from build123d import *
from OCP.BRepFilletAPI import BRepFilletAPI_MakeChamfer

# Parameters (mm, degrees)
EXTRUDE_1_DEPTH    = 2.4
HOLE_WIZARD_M3_1_D = 3.242
CHAMFER_1_SIZE     = 0.45
CHAMFER_1_SIZE_2   = 0.259807621
CHAMFER_3_SIZE     = 0.379


with BuildPart() as part:
    # 草圖1 → 填料-伸長1 (new body)
    with BuildSketch(Plane(origin=(0, 0, 0), x_dir=(0, -1, 0), z_dir=(-1, 0, 0))):
        with BuildLine():
            Line((-1.746239959, 2.975423668), (-3.449912463, 0.024576332))
            ThreePointArc((-3.449912463, 0.024576332), (-3.45, 0), (-3.449912463, -0.024576332))
            Line((-3.449912463, -0.024576332), (-1.746239959, -2.975423668))
            ThreePointArc((-1.746239959, -2.975423668), (-1.725, -2.987787643), (-1.703672504, -3))
            Line((-1.703672504, -3), (1.703672504, -3))
            ThreePointArc((1.703672504, -3), (1.725, -2.987787643), (1.746239959, -2.975423668))
            Line((1.746239959, -2.975423668), (3.449912463, -0.024576332))
            ThreePointArc((3.449912463, -0.024576332), (3.45, 0), (3.449912463, 0.024576332))
            Line((3.449912463, 0.024576332), (1.746239959, 2.975423668))
            ThreePointArc((1.746239959, 2.975423668), (1.725, 2.987787643), (1.703672504, 3))
            Line((1.703672504, 3), (-1.703672504, 3))
            ThreePointArc((-1.703672504, 3), (-1.725, 2.987787643), (-1.746239959, 2.975423668))
        make_face()
    extrude(amount=-EXTRUDE_1_DEPTH)

    # M3 餘隙孔1 (through all)
    with Locations(Plane(origin=(2.4, 0, 0), x_dir=(0, 0, -1), z_dir=(1, 0, 0))):
        with Locations((0, 0)):
            Hole(HOLE_WIZARD_M3_1_D / 2)

    # 導角1
    chamfer_1_edges_1 = [part.edges().sort_by_distance(p)[0] for p in [
        (0, -3.45, 0),
    ]]
    chamfer_1_side_1 = [part.faces().sort_by_distance(p)[0] for p in [
        (0, -3.444803848, 0),
    ]]
    chamfer_1_edges_2 = [part.edges().sort_by_distance(p)[0] for p in [
        (0, 1.725, 2.987787643),
    ]]
    chamfer_1_side_2 = [part.faces().sort_by_distance(p)[0] for p in [
        (0.005196152, 1.725, 2.987787643),
    ]]
    chamfer_1_edges_3 = [part.edges().sort_by_distance(p)[0] for p in [
        (0, 3.45, 0),
    ]]
    chamfer_1_side_3 = [part.faces().sort_by_distance(p)[0] for p in [
        (0, 3.444803848, 0),
    ]]
    chamfer_1_edges_4 = [part.edges().sort_by_distance(p)[0] for p in [
        (0, 1.725, -2.987787643),
    ]]
    chamfer_1_side_4 = [part.faces().sort_by_distance(p)[0] for p in [
        (0, 1.722401924, -2.983287643),
    ]]
    chamfer_1_edges_5 = [part.edges().sort_by_distance(p)[0] for p in [
        (0, -1.725, -2.987787643),
    ]]
    chamfer_1_side_5 = [part.faces().sort_by_distance(p)[0] for p in [
        (0, -1.722401924, -2.983287643),
    ]]
    chamfer_1_edges_6 = [part.edges().sort_by_distance(p)[0] for p in [
        (2.4, -1.725, 2.987787643),
    ]]
    chamfer_1_side_6 = [part.faces().sort_by_distance(p)[0] for p in [
        (2.4, -1.722401924, 2.983287643),
    ]]
    chamfer_1_edges_7 = [part.edges().sort_by_distance(p)[0] for p in [
        (2.4, 3.45, 0),
    ]]
    chamfer_1_side_7 = [part.faces().sort_by_distance(p)[0] for p in [
        (2.4, 3.444803848, 0),
    ]]
    chamfer_1 = BRepFilletAPI_MakeChamfer(part.part.solid().wrapped)
    for e in chamfer_1_edges_1:
        chamfer_1.Add(CHAMFER_1_SIZE - 0.0001, CHAMFER_1_SIZE_2 - 0.0001, e.wrapped, chamfer_1_side_1[0].wrapped)
    for e in chamfer_1_edges_2:
        chamfer_1.Add(CHAMFER_1_SIZE_2 - 0.0001, CHAMFER_1_SIZE - 0.0001, e.wrapped, chamfer_1_side_2[0].wrapped)
    for e in chamfer_1_edges_3:
        chamfer_1.Add(CHAMFER_1_SIZE - 0.0001, CHAMFER_1_SIZE_2 - 0.0001, e.wrapped, chamfer_1_side_3[0].wrapped)
    for e in chamfer_1_edges_4:
        chamfer_1.Add(CHAMFER_1_SIZE - 0.0001, CHAMFER_1_SIZE_2 - 0.0001, e.wrapped, chamfer_1_side_4[0].wrapped)
    for e in chamfer_1_edges_5:
        chamfer_1.Add(CHAMFER_1_SIZE - 0.0001, CHAMFER_1_SIZE_2 - 0.0001, e.wrapped, chamfer_1_side_5[0].wrapped)
    for e in chamfer_1_edges_6:
        chamfer_1.Add(CHAMFER_1_SIZE_2 - 0.0001, CHAMFER_1_SIZE - 0.0001, e.wrapped, chamfer_1_side_6[0].wrapped)
    for e in chamfer_1_edges_7:
        chamfer_1.Add(CHAMFER_1_SIZE_2 - 0.0001, CHAMFER_1_SIZE - 0.0001, e.wrapped, chamfer_1_side_7[0].wrapped)
    add(Compound.cast(chamfer_1.Shape()), mode=Mode.REPLACE)  # a hair under: the kernel refuses the full size

    # 導角3
    chamfer_3_edges = [part.edges().sort_by_distance(p)[0] for p in [
        (2.4, 0, -1.621),
        (0, 0, -1.621),
    ]]
    chamfer(chamfer_3_edges, length=CHAMFER_3_SIZE)


solid = part.part
Geometry: final body of the model. Coordinates: model frame, mm. Round coordinates to 2 decimals unless told otherwise and drop trailing zeros. Loops run counter-clockwise (first coordinate to the right, second up) from the corner with the lowest first, then second, coordinate; pieces in that order, holes last. Notation, with made-up numbers: M -0.75,29 L 24.25,29 A25 ccw 24.25,47 Z; hole C 33,43 d9. An arc over 180 degrees is marked long. Put each result on its own line as item: value. Start each with the question number.
(1) Contact query for flat-ended pins moving along their axis: pin 1 Ø1 at (x, z) = (2, 2.5) entering from -Y; pin 2 Ø1 at (x, y) = (1, -2.5) entering from +Z; pin 3 Ø2.5 at (y, z) = (0, 0) entering from +X. Output: stop coordinate, or through.
(2) Draft query along Y for faces 1 (the face through (1, 0, 3)), 2 (the face through (1.189, -1.438, 0.748)), 3 (the face through (0.102, -3.176, -0.008)). Return one class per face: +Y half, -Y half, draft (parallel to the pull), parting line (faces both ways), or undercut.
(3) Material intervals for line 1 along Y through (x, z) = (1.35, 0); line 2 along Y through (x, z) = (0.95, 1.4); line 3 along Z through (x, y) = (1.7, 2.25), sorted ascending. Write a range as [from, to].
(4) Section query A-A (x = 1.85). Return loops of the section in (y, z).
(5) Section query B-B (x = 2.2). Return loops of the section in (y, z), then the cut area to 3 significant figures.
Findings below:
1. pin 1: stops at y = -2.31
1. pin 2: stops at z = 2.54
1. pin 3: passes through
2. face 1: draft
2. face 2: undercut
2. face 3: -Y half
3. line 1: y = [-3.45, -1.62], [1.62, 3.45]
3. line 2: y = [-2.66, -0.82], [0.82, 2.66]
3. line 3: z = [-2.1, 2.1]
4. outline: M -3.45,-0.02 L -1.75,-2.98 A3.45 ccw -1.7,-3 L 1.7,-3 A3.45 ccw 1.75,-2.98 L 3.45,-0.02 A3.45 ccw 3.45,0.02 L 1.75,2.98 A3.45 ccw 1.7,3 L -1.7,3 A3.45 ccw -1.75,2.98 L -3.45,0.02 A3.45 ccw Z; hole C 0,0 d3.24
5. outline: M -3.45,-0.02 L -1.75,-2.98 A3.45 ccw -1.7,-3 L 1.7,-3 A3.45 ccw 1.75,-2.98 L 3.29,-0.3 A3.31 ccw 3.29,0.3 L 1.75,2.98 A3.45 ccw 1.7,3 L -1.39,3 A3.31 ccw -1.9,2.7 L -3.45,0.02 A3.45 ccw Z; hole C 0,0 d3.6
5. area: 20.9 mm2
